from build123d import *

# Parameters (mm, degrees)
SKETCH1_R               = 85
BOSS_EXTRUDE1_DEPTH     = 200
CUT_EXTRUDE1_DEPTH      = 234.345237792
CUT_EXTRUDE1_DEPTH_BACK = 234.345237792
SKETCH2_R               = 75
CUT_EXTRUDE3_DEPTH      = 234.34523795
CUT_EXTRUDE3_DEPTH_BACK = 234.34523795
SKETCH3_R               = 10
CUT_EXTRUDE4_DEPTH      = 234.34523795
CUT_EXTRUDE4_DEPTH_BACK = 234.34523795
SKETCH4_R               = 10


with BuildPart() as part:
    # Sketch1 → Boss-Extrude1 (new body)
    with BuildSketch(Plane.XY):
        Circle(SKETCH1_R)
    extrude(amount=BOSS_EXTRUDE1_DEPTH)

    # Sketch2 → Cut-Extrude1 (cut, two sides: drawn at the far end of the back side and taken through both)
    with BuildSketch(Plane(origin=(0, 0, 0), x_dir=(0, 0, -1), z_dir=(1, 0, 0)).offset(-CUT_EXTRUDE1_DEPTH_BACK)):
        Circle(SKETCH2_R)
    extrude(amount=CUT_EXTRUDE1_DEPTH + CUT_EXTRUDE1_DEPTH_BACK, mode=Mode.SUBTRACT)

    # Sketch3 → Cut-Extrude3 (cut, two sides: drawn at the far end of the back side and taken through both)
    with BuildSketch(Plane(origin=(0, 0, 0), x_dir=(1, 0, 0), z_dir=(0, 1, 0)).offset(-CUT_EXTRUDE3_DEPTH_BACK)):
        with Locations(Location((0, -20, 0), (0, 0, 270))):
            Circle(SKETCH3_R)
    extrude(amount=CUT_EXTRUDE3_DEPTH + CUT_EXTRUDE3_DEPTH_BACK, mode=Mode.SUBTRACT)

    # Sketch4 → Cut-Extrude4 (cut, two sides: drawn at the far end of the back side and taken through both)
    with BuildSketch(Plane.XY.offset(-CUT_EXTRUDE4_DEPTH_BACK)):
        Circle(SKETCH4_R)
    extrude(amount=CUT_EXTRUDE4_DEPTH + CUT_EXTRUDE4_DEPTH_BACK, mode=Mode.SUBTRACT)


solid = part.part
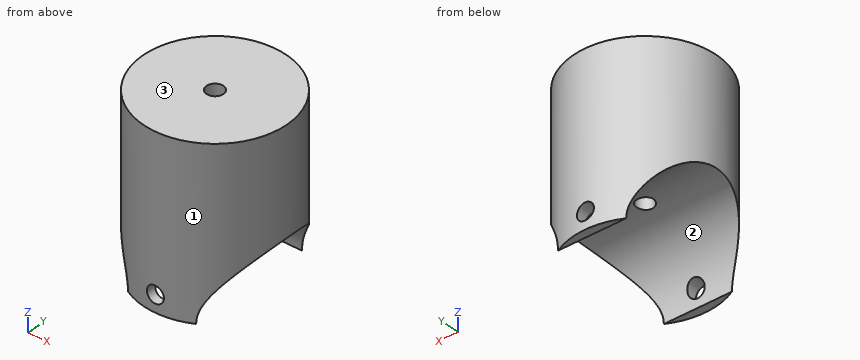
Here's how the part is built. I have some questions about the finished solid (model axes, mm). Face numbers are marked on the shaded views. Coordinates: 2 decimals unless noted, no trailing zeros. Order: outer loops, then holes, each group sorted by start corner. A loop starts at its lowest first (then second) coordinate and runs counter-clockwise, first axis right, second up.
Item 1: If we section it at A-A on y = 0: List the corners of the cut face in (x, z) for me.
Result sheet:
outline: (-85, 75) - (-10, 75) - (-10, 200) - (-85, 200) - close; (10, 75) - (85, 75) - (85, 200) - (10, 200) - close
Item 2: I need wall thicknesses on line 1 (Y direction, x = 0, z = 111); line 2 (Z direction, x = 0, y = 78); line 3 (Y direction, x = 8, z = 181.5). Which ranges of each line are inside material? Lowest first, please.
Result sheet:
line 1: y = -85 to -10, 10 to 85
line 2: z = 0 to 10, 30 to 200
line 3: y = -84.62 to -6, 6 to 84.62
Item 3: If we section it at B-B on z = 26: List the corners of the cut face in (x, y) for me, plus the area to 3 significant figures.
Result sheet:
outline: (-47.71, -70.35) arc R85 ccw to (-8, -84.62) - (-8, -70.35) - close; (-47.71, 70.35) - (-8, 70.35) - (-8, 84.62) arc R85 ccw to start; (8, -84.62) arc R85 ccw to (47.71, -70.35) - (8, -70.35) - close; (8, 70.35) - (47.71, 70.35) arc R85 ccw to (8, 84.62) - close
area: 1,430 mm2
Item 4: If we section it at D-D on z = 131: List the corners of the cut face in (x, y) for me.
Result sheet:
outline: circle Ø170 at (0, 0); hole circle Ø20 at (0, 0)
Item 5: If we mould it in two halves opening along Y, with no side actions, what happens to the marked faces 1, 2 and 3? For each: +Y half, -Y half, draft (parallel to the pull), parting line (faces both ways), or undercut.
Result sheet:
face 1: parting line
face 2: undercut
face 3: draft
Item 6: If we section it at C-C on x = 0: List the corners of the cut face in (y, z) for me, plus the area to 3 significant figures.
Result sheet:
outline: (-85, 0) - (-75, 0) arc R75 cw to (-74.33, 10) - (-85, 10) - close; (-85, 30) - (-68.74, 30) arc R75 cw to (-10, 74.33) - (-10, 200) - (-85, 200) - close; (10, 74.33) arc R75 cw to (68.74, 30) - (85, 30) - (85, 200) - (10, 200) - close; (74.33, 10) arc R75 cw to (75, 0) - (85, 0) - (85, 10) - close
area: 22,100 mm2
Item 7: For P1, Ø12, axis at x = 0, z = 20, coming from the +Y side; P2, Ø3, axis at x = -2, z = 146.5, coming from the +Y side; P3, Ø5, axis at x = -24.5, z = 50.5, coming from the +Y side; P4, Ø10, axis at y = -45, z = 73, coming from the +X side, each with a flat end and sliding along its axis, tell me the tip position at first contact or that it passes through.
Result sheet:
P1: passes through
P2: stops at y = 85
P3: stops at y = 82.1
P4: stops at x = 75
